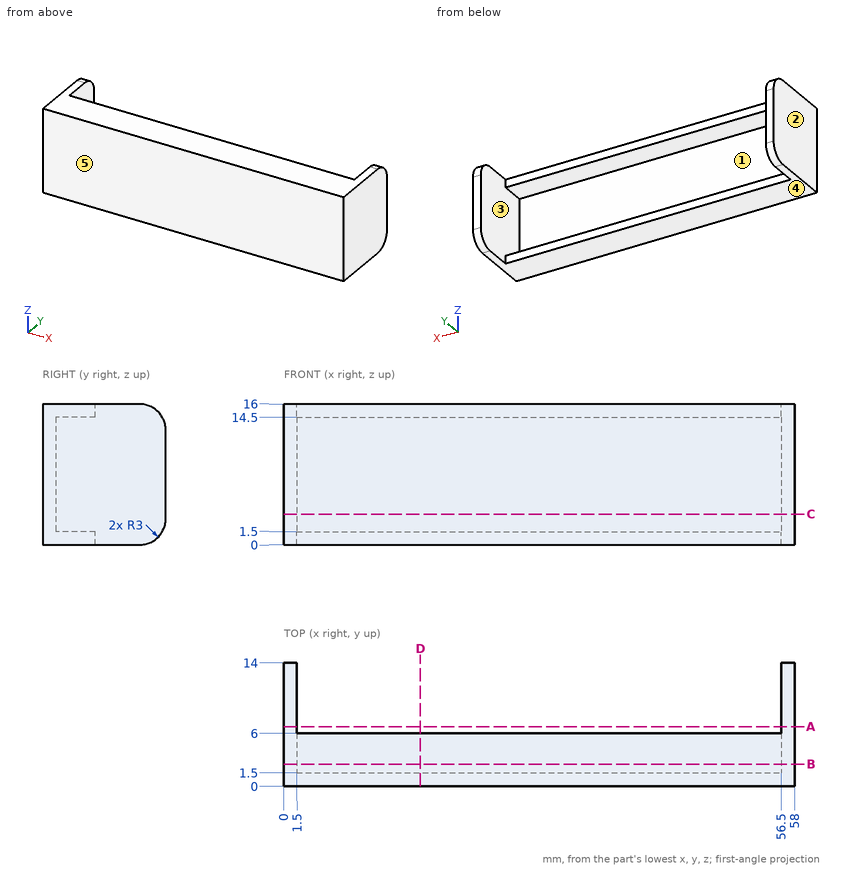
For this review, use the dimensioned drawing (mm, ordinates from the lowest corner) and the shaded views. A direction names the side the tool comes from. Round coordinates to 2 decimals unless told otherwise and drop trailing zeros. Write each loop counter-clockwise with the first axis right and the second up, starting at its lowest first coordinate (ties: lowest second). Pieces come first, ordered by that corner, then holes. Notation, with made-up numbers: (73, 18.5) -> (104, 18.5) arc R25 cw to (104, 44.5) -> close; hole circle Ø5 at (21, 28.25). An arc over 180 degrees is marked (long way). Answer in a Markdown table with one row per item.
Q1. Clearance check with flat-ended pins moving along their axes: pin 1 Ø1.2 at (x, z) = (18, 1) entering from +Y; pin 2 Ø6 at (x, y) = (35.5, 10.5) entering from +Z; pin 3 Ø5 at (x, z) = (33, 11) entering from +Y. State where each tip first meets the part, or that it passes through.
The answers:
| item | result |
|---|---|
| pin 1 | y = 6 |
| pin 2 | through |
| pin 3 | y = 1.5 |
Q2. Take a section at C-C, the plane z = 3.5. State the section outline as (x, y) points, then the cut area to 4 significant figures.
The answers:
| item | result |
|---|---|
| outline | (0, 0) -> (58, 0) -> (58, 14) -> (56.5, 14) -> (56.5, 1.5) -> (1.5, 1.5) -> (1.5, 14) -> (0, 14) -> close |
| area | 124.5 mm² |
Q3. Take a section at B-B, the plane y = 2.5. State the section outline as (x, z) points, then the cut area to 3 significant figures.
The answers:
| item | result |
|---|---|
| outline | (0, 0) -> (58, 0) -> (58, 16) -> (0, 16) -> close; hole (1.5, 1.5) -> (56.5, 1.5) -> (56.5, 14.5) -> (1.5, 14.5) -> close |
| area | 213 mm² |
Q4. Draft analysis for pull direction Z (two halves, no side actions). For the marked faces 3, 4 and 5, state which applies: +Z half, -Z half, draft (parallel to the pull), parting line (faces both ways), or undercut.
The answers:
| item | result |
|---|---|
| face 3 | undercut |
| face 4 | -Z half |
| face 5 | draft |
Q5. Take a section at D-D, the plane x = 15.5. State the section outline as (y, z) points, then the cut area to 3 significant figures.
The answers:
| item | result |
|---|---|
| outline | (0, 0) -> (6, 0) -> (6, 1.5) -> (1.5, 1.5) -> (1.5, 14.5) -> (6, 14.5) -> (6, 16) -> (0, 16) -> close |
| area | 37.5 mm² |
Q6. To check wall thickness, follow L1, parallel to Z at x = 27.5, y = 3; L2, parallel to X at y = 6.5, z = 12; L3, parallel to Y at x = 28.5, z = 9. State the ranges of each line that lie inside material, in increasing order. Write a range as [from, to].
The answers:
| item | result |
|---|---|
| L1 | [0, 1.5], [14.5, 16] |
| L2 | [0, 1.5], [56.5, 58] |
| L3 | [0, 1.5] |
Q7. Take a section at A-A, the plane y = 6.75. State the section outline as (x, z) points, then the cut area to 3 significant figures.
The answers:
| item | result |
|---|---|
| outline | (0, 0) -> (1.5, 0) -> (1.5, 16) -> (0, 16) -> close; (56.5, 0) -> (58, 0) -> (58, 16) -> (56.5, 16) -> close |
| area | 48.0 mm² |
Q8. For the marked faces 1 and 2, list the 3-axis set-ups (+Z, -Z, +X, -X, +Y, -Y) from which the entire face can be reached by the end or side of a thin tool; tool diameter is ignored.
The answers:
| item | result |
|---|---|
| face 1 | +Y |
| face 2 | +Z, -Z, -X, +Y, -Y |
